```python
from build123d import *

# Parameters (mm, degrees)
SKETCH1_R           = 2.4511
BOSS_EXTRUDE1_DEPTH = 4.7625


with BuildPart() as part:
    # Sketch1 → Boss-Extrude1 (new, symmetric)
    with BuildSketch(Plane(origin=(0, 0, 0), x_dir=(1, 0, 0), z_dir=(0, 1, 0))):
        with BuildLine():
            ThreePointArc((-1.850768, -6.777037356), (-1.816941892, -6.962421006), (-1.663291889, -7.071521784))
            ThreePointArc((-1.663291889, -7.071521784), (-1.417233644, -7.124914669), (-1.169472895, -7.169748489))
            ThreePointArc((-1.169472895, -7.169748489), (-0.985767742, -7.127751824), (-0.883573242, -6.969424355))
            ThreePointArc((-0.883573242, -6.969424355), (-0.839120956, -6.792881518), (-0.773880597, -6.622919538))
            ThreePointArc((-0.773880597, -6.622919538), (0, -6.1245), (0.773880597, -6.622919538))
            ThreePointArc((0.773880597, -6.622919538), (0.839120956, -6.792881518), (0.883573242, -6.969424355))
            ThreePointArc((0.883573242, -6.969424355), (0.985767742, -7.127751824), (1.169472895, -7.169748489))
            ThreePointArc((1.169472895, -7.169748489), (1.417233644, -7.124914669), (1.663291889, -7.071521784))
            ThreePointArc((1.663291889, -7.071521784), (1.816941892, -6.962421006), (1.850768, -6.777037356))
            ThreePointArc((1.850768, -6.777037356), (1.824276538, -6.596921889), (1.819509137, -6.414931089))
            ThreePointArc((1.819509137, -6.414931089), (2.343744682, -5.658300197), (3.249454025, -5.822628523))
            ThreePointArc((3.249454025, -5.822628523), (3.374769892, -5.954686513), (3.483398468, -6.100779674))
            ThreePointArc((3.483398468, -6.100779674), (3.638403174, -6.20794704), (3.824196033, -6.176445981))
            ThreePointArc((3.824196033, -6.176445981), (4.035939958, -6.040210999), (4.242835561, -5.896719991))
            ThreePointArc((4.242835561, -5.896719991), (4.343038594, -5.737124705), (4.303346591, -5.552907854))
            ThreePointArc((4.303346591, -5.552907854), (4.209944466, -5.396640704), (4.135895098, -5.230327534))
            ThreePointArc((4.135895098, -5.230327534), (4.330675481, -4.330675481), (5.230327534, -4.135895098))
            ThreePointArc((5.230327534, -4.135895098), (5.396640704, -4.209944466), (5.552907854, -4.303346591))
            ThreePointArc((5.552907854, -4.303346591), (5.737124705, -4.343038594), (5.896719991, -4.242835561))
            ThreePointArc((5.896719991, -4.242835561), (6.040210999, -4.035939958), (6.176445981, -3.824196033))
            ThreePointArc((6.176445981, -3.824196033), (6.20794704, -3.638403174), (6.100779674, -3.483398468))
            ThreePointArc((6.100779674, -3.483398468), (5.954686513, -3.374769892), (5.822628523, -3.249454025))
            ThreePointArc((5.822628523, -3.249454025), (5.658300197, -2.343744682), (6.414931089, -1.819509137))
            ThreePointArc((6.414931089, -1.819509137), (6.596921889, -1.824276538), (6.777037356, -1.850768))
            ThreePointArc((6.777037356, -1.850768), (6.962421006, -1.816941892), (7.071521784, -1.663291889))
            ThreePointArc((7.071521784, -1.663291889), (7.124914669, -1.417233644), (7.169748489, -1.169472895))
            ThreePointArc((7.169748489, -1.169472895), (7.127751824, -0.985767742), (6.969424355, -0.883573242))
            ThreePointArc((6.969424355, -0.883573242), (6.792881518, -0.839120956), (6.622919538, -0.773880597))
            ThreePointArc((6.622919538, -0.773880597), (6.1245, 0), (6.622919538, 0.773880597))
            ThreePointArc((6.622919538, 0.773880597), (6.792881518, 0.839120956), (6.969424355, 0.883573242))
            ThreePointArc((6.969424355, 0.883573242), (7.127751824, 0.985767742), (7.169748489, 1.169472895))
            ThreePointArc((7.169748489, 1.169472895), (7.124914669, 1.417233644), (7.071521784, 1.663291889))
            ThreePointArc((7.071521784, 1.663291889), (6.962421006, 1.816941892), (6.777037356, 1.850768))
            ThreePointArc((6.777037356, 1.850768), (6.596921889, 1.824276538), (6.414931089, 1.819509137))
            ThreePointArc((6.414931089, 1.819509137), (5.658300197, 2.343744682), (5.822628523, 3.249454025))
            ThreePointArc((5.822628523, 3.249454025), (5.954686513, 3.374769892), (6.100779674, 3.483398468))
            ThreePointArc((6.100779674, 3.483398468), (6.20794704, 3.638403174), (6.176445981, 3.824196033))
            ThreePointArc((6.176445981, 3.824196033), (6.040210999, 4.035939958), (5.896719991, 4.242835561))
            ThreePointArc((5.896719991, 4.242835561), (5.737124705, 4.343038594), (5.552907854, 4.303346591))
            ThreePointArc((5.552907854, 4.303346591), (5.396640704, 4.209944466), (5.230327534, 4.135895098))
            ThreePointArc((5.230327534, 4.135895098), (4.330675481, 4.330675481), (4.135895098, 5.230327534))
            ThreePointArc((4.135895098, 5.230327534), (4.209944466, 5.396640704), (4.303346591, 5.552907854))
            ThreePointArc((4.303346591, 5.552907854), (4.343038594, 5.737124705), (4.242835561, 5.896719991))
            ThreePointArc((4.242835561, 5.896719991), (4.035939958, 6.040210999), (3.824196033, 6.176445981))
            ThreePointArc((3.824196033, 6.176445981), (3.638403174, 6.20794704), (3.483398468, 6.100779674))
            ThreePointArc((3.483398468, 6.100779674), (3.374769892, 5.954686513), (3.249454025, 5.822628523))
            ThreePointArc((3.249454025, 5.822628523), (2.343744682, 5.658300197), (1.819509137, 6.414931089))
            ThreePointArc((1.819509137, 6.414931089), (1.824276538, 6.596921889), (1.850768, 6.777037356))
            ThreePointArc((1.850768, 6.777037356), (1.816941892, 6.962421006), (1.663291889, 7.071521784))
            ThreePointArc((1.663291889, 7.071521784), (1.417233644, 7.124914669), (1.169472895, 7.169748489))
            ThreePointArc((1.169472895, 7.169748489), (0.985767742, 7.127751824), (0.883573242, 6.969424355))
            ThreePointArc((0.883573242, 6.969424355), (0.839120956, 6.792881518), (0.773880597, 6.622919538))
            ThreePointArc((0.773880597, 6.622919538), (0, 6.1245), (-0.773880597, 6.622919538))
            ThreePointArc((-0.773880597, 6.622919538), (-0.839120956, 6.792881518), (-0.883573242, 6.969424355))
            ThreePointArc((-0.883573242, 6.969424355), (-0.985767742, 7.127751824), (-1.169472895, 7.169748489))
            ThreePointArc((-1.169472895, 7.169748489), (-1.417233644, 7.124914669), (-1.663291889, 7.071521784))
            ThreePointArc((-1.663291889, 7.071521784), (-1.816941892, 6.962421006), (-1.850768, 6.777037356))
            ThreePointArc((-1.850768, 6.777037356), (-1.824276538, 6.596921889), (-1.819509137, 6.414931089))
            ThreePointArc((-1.819509137, 6.414931089), (-2.343744682, 5.658300197), (-3.249454025, 5.822628523))
            ThreePointArc((-3.249454025, 5.822628523), (-3.374769892, 5.954686513), (-3.483398468, 6.100779674))
            ThreePointArc((-3.483398468, 6.100779674), (-3.638403174, 6.20794704), (-3.824196033, 6.176445981))
            ThreePointArc((-3.824196033, 6.176445981), (-4.035939958, 6.040210999), (-4.242835561, 5.896719991))
            ThreePointArc((-4.242835561, 5.896719991), (-4.343038594, 5.737124705), (-4.303346591, 5.552907854))
            ThreePointArc((-4.303346591, 5.552907854), (-4.209944466, 5.396640704), (-4.135895098, 5.230327534))
            ThreePointArc((-4.135895098, 5.230327534), (-4.330675481, 4.330675481), (-5.230327534, 4.135895098))
            ThreePointArc((-5.230327534, 4.135895098), (-5.396640704, 4.209944466), (-5.552907854, 4.303346591))
            ThreePointArc((-5.552907854, 4.303346591), (-5.737124705, 4.343038594), (-5.896719991, 4.242835561))
            ThreePointArc((-5.896719991, 4.242835561), (-6.040210999, 4.035939958), (-6.176445981, 3.824196033))
            ThreePointArc((-6.176445981, 3.824196033), (-6.20794704, 3.638403174), (-6.100779674, 3.483398468))
            ThreePointArc((-6.100779674, 3.483398468), (-5.954686513, 3.374769892), (-5.822628523, 3.249454025))
            ThreePointArc((-5.822628523, 3.249454025), (-5.658300197, 2.343744682), (-6.414931089, 1.819509137))
            ThreePointArc((-6.414931089, 1.819509137), (-6.596921889, 1.824276538), (-6.777037356, 1.850768))
            ThreePointArc((-6.777037356, 1.850768), (-6.962421006, 1.816941892), (-7.071521784, 1.663291889))
            ThreePointArc((-7.071521784, 1.663291889), (-7.124914669, 1.417233644), (-7.169748489, 1.169472895))
            ThreePointArc((-7.169748489, 1.169472895), (-7.127751824, 0.985767742), (-6.969424355, 0.883573242))
            ThreePointArc((-6.969424355, 0.883573242), (-6.792881518, 0.839120956), (-6.622919538, 0.773880597))
            ThreePointArc((-6.622919538, 0.773880597), (-6.1245, 0), (-6.622919538, -0.773880597))
            ThreePointArc((-6.622919538, -0.773880597), (-6.792881518, -0.839120956), (-6.969424355, -0.883573242))
            ThreePointArc((-6.969424355, -0.883573242), (-7.127751824, -0.985767742), (-7.169748489, -1.169472895))
            ThreePointArc((-7.169748489, -1.169472895), (-7.124914669, -1.417233644), (-7.071521784, -1.663291889))
            ThreePointArc((-7.071521784, -1.663291889), (-6.962421006, -1.816941892), (-6.777037356, -1.850768))
            ThreePointArc((-6.777037356, -1.850768), (-6.596921889, -1.824276538), (-6.414931089, -1.819509137))
            ThreePointArc((-6.414931089, -1.819509137), (-5.658300197, -2.343744682), (-5.822628523, -3.249454025))
            ThreePointArc((-5.822628523, -3.249454025), (-5.954686513, -3.374769892), (-6.100779674, -3.483398468))
            ThreePointArc((-6.100779674, -3.483398468), (-6.20794704, -3.638403174), (-6.176445981, -3.824196033))
            ThreePointArc((-6.176445981, -3.824196033), (-6.040210999, -4.035939958), (-5.896719991, -4.242835561))
            ThreePointArc((-5.896719991, -4.242835561), (-5.737124705, -4.343038594), (-5.552907854, -4.303346591))
            ThreePointArc((-5.552907854, -4.303346591), (-5.396640704, -4.209944466), (-5.230327534, -4.135895098))
            ThreePointArc((-5.230327534, -4.135895098), (-4.330675481, -4.330675481), (-4.135895098, -5.230327534))
            ThreePointArc((-4.135895098, -5.230327534), (-4.209944466, -5.396640704), (-4.303346591, -5.552907854))
            ThreePointArc((-4.303346591, -5.552907854), (-4.343038594, -5.737124705), (-4.242835561, -5.896719991))
            ThreePointArc((-4.242835561, -5.896719991), (-4.035939958, -6.040210999), (-3.824196033, -6.176445981))
            ThreePointArc((-3.824196033, -6.176445981), (-3.638403174, -6.20794704), (-3.483398468, -6.100779674))
            ThreePointArc((-3.483398468, -6.100779674), (-3.374769892, -5.954686513), (-3.249454025, -5.822628523))
            ThreePointArc((-3.249454025, -5.822628523), (-2.343744682, -5.658300197), (-1.819509137, -6.414931089))
            ThreePointArc((-1.819509137, -6.414931089), (-1.824276538, -6.596921889), (-1.850768, -6.777037356))
        make_face()
        with Locations(Location((0, 0, 0), (0, 0, 90))):
            Circle(SKETCH1_R, mode=Mode.SUBTRACT)
    extrude(amount=BOSS_EXTRUDE1_DEPTH, both=True)


solid = part.part
```
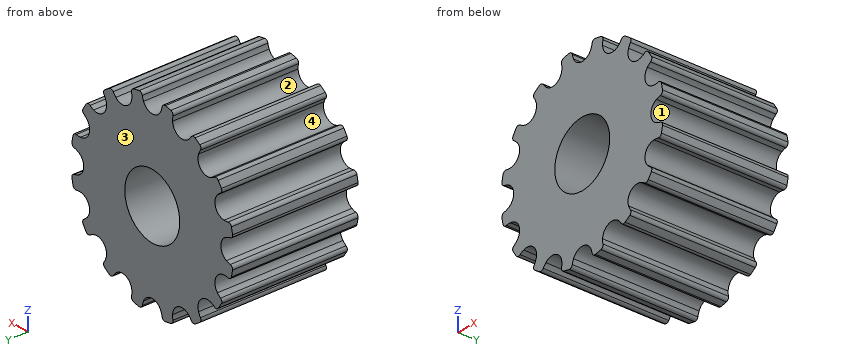
Input: part model. Units: mm. Frame: model coordinates. Face numbers are marked on the shaded views. Give positions to 0.01 mm unless a question says otherwise; leave off trailing zeros. Order: outer loops, then holes, each group sorted by start corner. A loop starts at its lowest first (then second) coordinate and runs counter-clockwise, first axis right, second up. Notation, with made-up numbers: M -18,85 L -6,85 A25 ccw -6,105 Z; hole C -24,-35.75 d1. An arc over 180 degrees is marked long. One line per question, with ' | ' between items. Start each with the question number.
1. Material intervals for probe 1 along X at (y, z) = (2.5, 0); probe 2 along X at (y, z) = (4, -4.25); probe 3 along X at (y, z) = (0.5, -5.75), sorted ascending. Write a range as [from, to].
2. First-contact query: pin 1 Ø1 at (y, z) = (3, 2.5) entering from +X. Flat tip, straight axial feed; report the tip coordinate or a pass-through.
3. Section query A-A (x = 0). Return the cut outline in (y, z).
4. Section query C-C (z = -3). Return the cut outline in (x, y), and give its area (3 significant figures).
5. Section query B-B (z = 0). Return the cut outline in (x, y).
6. Pull-direction query (X, two-part tool) for the marked faces 1, 2, 3 and 4; classes: released by +X, released by -X, zero draft, split by the parting line, or undercut.
Here are the results:
1) probe 1: [-6.12, -2.45], [2.45, 6.12] | probe 2: [-5.89, -5.47], [-4.42, 4.42], [5.47, 5.89] | probe 3: [-4.34, -3.16], [-2.18, 2.18], [3.16, 4.34]
2) pin 1: x = 5.92
3) outline: M -4.76,-6.12 L 4.76,-6.12 L 4.76,-2.45 L -4.76,-2.45 Z; M -4.76,2.45 L 4.76,2.45 L 4.76,6.12 L -4.76,6.12 Z
4) outline: M -5.66,-4.76 L 5.66,-4.76 L 5.66,4.76 L -5.66,4.76 Z | area: 108 mm²
5) outline: M -6.12,-4.76 L -2.45,-4.76 L -2.45,4.76 L -6.12,4.76 Z; M 2.45,-4.76 L 6.12,-4.76 L 6.12,4.76 L 2.45,4.76 Z
6) face 1: released by +X | face 2: undercut | face 3: zero draft | face 4: undercut
